Verification items for the finished model (mm, model axes). Face numbers are marked on the shaded views. A direction names the side the tool comes from. Coordinates: 2 decimals unless noted, no trailing zeros. Write each loop counter-clockwise with the first axis right and the second up, starting at its lowest first coordinate (ties: lowest second). Pieces come first, ordered by that corner, then holes. Notation, with made-up numbers: M -22,-5 L -2,-5 A6 cw -2,-1 Z; hole C -15.5,-22 d9. An arc over 180 degrees is marked long. Answer in a Markdown table with one row per item.
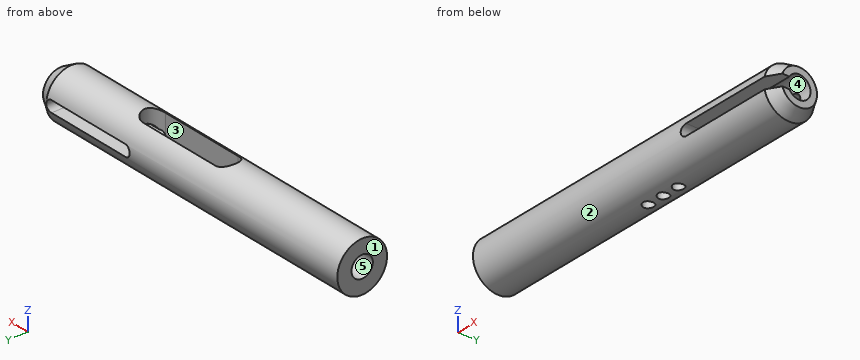
from build123d import *

# Parameters (mm, degrees)
F0_R           = 7
F1_DEPTH       = 100
F2_R           = 3.175
F3_DEPTH       = 35
F4_R           = 3
F5_DEPTH       = 25
F6_SIZE2       = 3.4641016151
F6_SIZE        = 2
F8_DEPTH       = 7.001
F8_DEPTH_BACK  = 1
F10_DEPTH      = 7.0010001
F10_DEPTH_BACK = 7.0010001
F11_W          = 15
F11_H          = 3.175
F12_DEPTH      = 25.0000003725
F13_R          = 1.5
F14_DEPTH      = 6.0010001


with BuildPart() as f1:
    # F0 (on Right) → F1 (new body)
    with BuildSketch(Plane.YZ):
        Circle(F0_R)
    extrude(amount=F1_DEPTH)

    # F2 (on face) → F3 (cut)
    with BuildSketch(Plane.YZ.offset(100)):
        Circle(F2_R)
    extrude(amount=-F3_DEPTH, mode=Mode.SUBTRACT)

    # F4 (on face) → F5 (cut)
    with BuildSketch(Plane(origin=(0, 0, 0), x_dir=(0, -1, 0), z_dir=(-1, 0, 0))):
        Circle(F4_R)
    extrude(amount=-F5_DEPTH, mode=Mode.SUBTRACT)

    # F6
    f6_edges = [f1.edges().sort_by_distance(p)[0] for p in [
        (100, -7, 0),
    ]]
    f6_side = f1.faces().sort_by_distance((100, -6.80201, 0))[0]
    chamfer(f6_edges, length=F6_SIZE, length2=F6_SIZE2, reference=f6_side)

    # F7 (on Top) → F8 (cut, two sides)
    with BuildSketch(Plane.XY) as f8_sk:
        with BuildLine():
            Line((69, 3.175), (45, 3.175))
            ThreePointArc((45, 3.175), (41.825, 0), (45, -3.175))
            Line((45, -3.175), (69, -3.175))
            ThreePointArc((69, -3.175), (72.175, 0), (69, 3.175))
        make_face()
    extrude(amount=F8_DEPTH, mode=Mode.SUBTRACT)
    extrude(f8_sk.sketch, amount=-F8_DEPTH_BACK, mode=Mode.SUBTRACT)

    # F9 (on Front) → F10 (cut, two sides)
    with BuildSketch(Plane.XZ) as f10_sk:
        with BuildLine():
            Line((95, 1.5875), (70.5, 1.5875))
            ThreePointArc((70.5, 1.5875), (68.9125, 0), (70.5, -1.5875))
            Line((70.5, -1.5875), (95, -1.5875))
            ThreePointArc((95, -1.5875), (96.5875, 0), (95, 1.5875))
        make_face()
    extrude(amount=-F10_DEPTH, mode=Mode.SUBTRACT)
    extrude(f10_sk.sketch, amount=F10_DEPTH_BACK, mode=Mode.SUBTRACT)

    # F11 (on Front) → F12 (cut)
    with BuildSketch(Plane.XZ):
        with Locations((95.5, 0)):
            Rectangle(F11_W, F11_H)
    extrude(amount=F12_DEPTH, mode=Mode.SUBTRACT)

    # F13 (on face) → F14 (cut, through all)
    with BuildSketch(Plane.XY.offset(-1)):
        with Locations((50, 0)):
            Circle(F13_R)
        with Locations((55, 0)):
            Circle(F13_R)
        with Locations((60, 0)):
            Circle(F13_R)
    extrude(amount=-F14_DEPTH, mode=Mode.SUBTRACT)


solid = f1.part
1) Sectioned sample at A-A (y = 0). Give the number of separate pieces and of enclosed holes in the cut face, then the cut area to 3 significant figures.
Response values:
| item | result |
|---|---|
| separate pieces | 5 |
| enclosed holes | 0 |
| area | 754 mm² |
2) Tool access check on the marked faces 4 and 5. Record the directions out of +Z, -Z, +X, -X, +Y, -Y that give a thin tool (end or side, any length) a straight path to the whole face; none if there is none.
Response values:
| item | result |
|---|---|
| face 4 | +X |
| face 5 | -X |
3) Sectioned sample at C-C (x = 50). Record the cut outline in (y, z) (3 decimals).
Response values:
| item | result |
|---|---|
| outline | M -3.175,-1 L -3.175,6.239 A7 ccw -1.5,-6.837 L -1.5,-1 Z; M 1.5,-6.837 A7 ccw 3.175,6.239 L 3.175,-1 L 1.5,-1 Z |
4) Thickness scan on L1, parallel to X at y = 0, z = -4.25; L2, parallel to X at y = 0.25, z = -1.75; L3, parallel to Z at x = 52.5, y = 6.25. Record the ranges inside material, lowest first. Write a range as [from, to].
Response values:
| item | result |
|---|---|
| L1 | x = [0, 48.5], [51.5, 53.5], [56.5, 58.5], [61.5, 100] |
| L2 | x = [25, 48.52], [51.48, 53.52], [56.48, 58.52], [61.48, 65] |
| L3 | z = [-3.15, 3.15] |
5) Depth check by flat-ended pin: pin 1 (2 mm diameter, centred on x = 85.5, y = 4.5, fed in from +Z); pin 2 (1 mm diameter, centred on y = -0.5, z = 2, fed in from +X); pin 3 (7 mm diameter, centred on y = 0, z = 0, fed in from -X); pin 4 (2.5 mm diameter, centred on y = -0.5, z = -1.5, fed in from +X). Enter the tip coordinate at first touch or a pass-through.
Response values:
| item | result |
|---|---|
| pin 1 | stops at z = 6.06 |
| pin 2 | stops at x = 41.99 |
| pin 3 | stops at x = 0 |
| pin 4 | stops at x = 65 |
6) Release check for a two-part mould opening along X. For the marked faces 1, 2 and 3 record: +X half, -X half, draft (parallel to the pull), parting line (faces both ways), or undercut.
Response values:
| item | result |
|---|---|
| face 1 | -X half |
| face 2 | draft |
| face 3 | undercut |
